Geometry: final body of the model. Coordinates: model frame, mm. Give positions to 0.01 mm unless a question says otherwise; leave off trailing zeros.
Q1. Draft query along X for faces 1 (the face through (27.783, -21.709, 2.958)), 2 (the face through (-111.983, -20, 3)), 3 (the face through (-1, -11, 6)), 4 (the face through (110.55, -27.08, 2.96)). Return one class per face: pulls with the +X half, pulls with the -X half, needs draft (parallel to the pull), parting line crosses it, or undercut.
Q2. Line query: L1, parallel to Y at x = 52, z = 3.3; L2, parallel to Y at x = 49.5, z = 4.25; L3, parallel to X at y = -25.5, z = 0.65. Output: solid intervals per line, ascending.
Q3. Cut plane A-A on z = 4.1. Count the separate pieces of the cut face and the enclosed holes in it, plus the area to 3 significant figures.
```python
from build123d import *

# Parameters (mm, degrees)
SKETCH1_W           = 225
SKETCH1_H           = 20
SKETCH1_R           = 3.75
SKETCH1_R_2         = 5.177315147
SKETCH1_R_3         = 5.175
SKETCH1_R_4         = 3.445800431
SKETCH1_R_5         = 7.5
BOSS_EXTRUDE1_DEPTH = 6
CHAMFER1_SIZE       = 5


with BuildPart() as part:
    # Sketch1 → Boss-Extrude1 (new body)
    with BuildSketch(Plane.XY):
        with Locations((0.517233183, -19.612075113)):
            Rectangle(SKETCH1_W, SKETCH1_H)
        with Locations((84.017233183, -19.612075113)):
            Circle(SKETCH1_R, mode=Mode.SUBTRACT)
        with Locations((52.017233183, -19.612075113)):
            Circle(SKETCH1_R, mode=Mode.SUBTRACT)
        with Locations((68.017233183, -19.612075113)):
            Circle(SKETCH1_R_2, mode=Mode.SUBTRACT)
        with Locations((-50.982766817, -19.612075113)):
            Circle(SKETCH1_R, mode=Mode.SUBTRACT)
        with Locations((-82.982766817, -19.612075113)):
            Circle(SKETCH1_R, mode=Mode.SUBTRACT)
        with Locations((-66.982766817, -19.612075113)):
            Circle(SKETCH1_R_3, mode=Mode.SUBTRACT)
        with Locations((30.517233183, -19.612075113)):
            Circle(SKETCH1_R_4, mode=Mode.SUBTRACT)
        with Locations((-29.482766817, -19.612075113)):
            Circle(SKETCH1_R_4, mode=Mode.SUBTRACT)
        with Locations((100.517233183, -19.612075113)):
            Circle(SKETCH1_R_4, mode=Mode.SUBTRACT)
        with Locations((-99.482766817, -19.612075113)):
            Circle(SKETCH1_R_4, mode=Mode.SUBTRACT)
        with Locations((0.517233183, -19.612075113)):
            Circle(SKETCH1_R_5, mode=Mode.SUBTRACT)
    extrude(amount=BOSS_EXTRUDE1_DEPTH)

    # Chamfer1
    chamfer1_edges = [part.edges().sort_by_distance(p)[0] for p in [
        (-111.982766817, -9.612075113, 3),
        (113.017233183, -9.612075113, 3),
        (113.017233183, -29.612075113, 3),
        (-111.982766817, -29.612075113, 3),
    ]]
    chamfer(chamfer1_edges, length=CHAMFER1_SIZE)


solid = part.part
```
Data:
1. face 1: undercut
1. face 2: pulls with the -X half
1. face 3: needs draft
1. face 4: pulls with the +X half
2. L1: y = -29.61 to -23.36, -15.86 to -9.61
2. L2: y = -29.61 to -22.39, -16.83 to -9.61
2. L3: x = -111.09 to -4.13, 5.16 to 112.13
3. separate pieces: 1
3. enclosed holes: 11
3. area: 3,780 mm2
